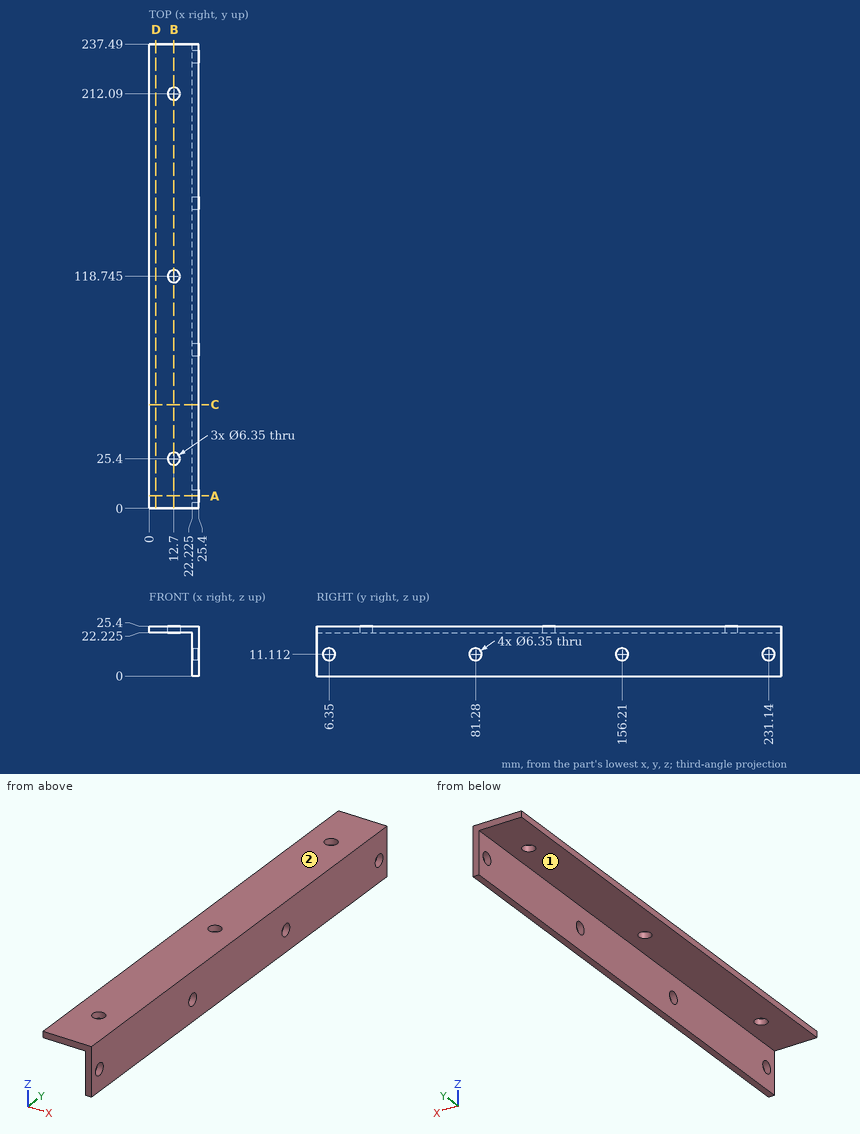
Verification items for this drawing (mm, ordinates from the low corner). A direction names the side the tool comes from. Coordinates: 2 decimals unless noted, no trailing zeros. Write each loop counter-clockwise with the first axis right and the second up, starting at its lowest first coordinate (ties: lowest second). Pieces come first, ordered by that corner, then holes. Notation, with made-up numbers: (-36, -17.75) -> (-18, -17.75) arc R8 ccw to (-18, -3.75) -> close; hole circle Ø10 at (4.5, -13). An arc over 180 degrees is marked (long way). One line per item, written item: value. Start each with the question number.
Q1. Cross-section at B-B on x = 12.7. Enter the section's corners in (y, z) (1 decimal).
Q2. Cross-section at D-D on x = 3.5. Enter the section's corners in (y, z) (1 decimal).
Q3. Access from +Z, -Z, +X, -X, +Y, -Y to the whole of each face (thin tool, end or side, straight path). Record for the marked faces 1 and 2.
Q4. Go/stop test with flat-tipped pins: P1, Ø12, axis at y = 142.5, z = 21, coming from the -X side; P2, Ø10, axis at y = 81.28, z = 11.11, coming from the -X side (1 decimal); P3, Ø1.5, axis at x = 6, y = 48.5, coming from the -Z side (1 decimal). Record where each tip stops, or that it passes through.
Q5. Thickness scan on L1, parallel to Y at x = 12.7, z = 23.85 (1 decimal); L2, parallel to Z at x = 24.05, y = 156.21; L3, parallel to X at y = 62, z = 14.25 (1 decimal). Record the ranges inside material, lowest first. Write a range as from..to.
Q6. Cross-section at A-A on y = 6.35. Enter the section's corners in (x, z) (1 decimal), and give its area (3 significant figures).
Q7. Cross-section at C-C on y = 53. Enter the section's corners in (x, z) (1 decimal), and give its area (3 significant figures).
Checked values:
1. outline: (0, 22.2) -> (22.2, 22.2) -> (22.2, 25.4) -> (0, 25.4) -> close; (28.6, 22.2) -> (115.6, 22.2) -> (115.6, 25.4) -> (28.6, 25.4) -> close; (121.9, 22.2) -> (208.9, 22.2) -> (208.9, 25.4) -> (121.9, 25.4) -> close; (215.3, 22.2) -> (237.5, 22.2) -> (237.5, 25.4) -> (215.3, 25.4) -> close
2. outline: (0, 22.2) -> (237.5, 22.2) -> (237.5, 25.4) -> (0, 25.4) -> close
3. face 1: -Z, -X, +Y, -Y
3. face 2: +Z, +X, -X, +Y, -Y
4. P1: stops at x = 0
4. P2: stops at x = 22.2
4. P3: stops at z = 22.2
5. L1: y = 0..22.2, 28.6..115.6, 121.9..208.9, 215.3..237.5
5. L2: z = 0..7.94, 14.29..25.4
5. L3: x = 22.2..25.4
6. outline: (0, 22.2) -> (22.2, 22.2) -> (22.2, 14.3) -> (25.4, 14.3) -> (25.4, 25.4) -> (0, 25.4) -> close; (22.2, 0) -> (25.4, 0) -> (25.4, 7.9) -> (22.2, 7.9) -> close
6. area: 131 mm²
7. outline: (0, 22.2) -> (22.2, 22.2) -> (22.2, 0) -> (25.4, 0) -> (25.4, 25.4) -> (0, 25.4) -> close
7. area: 151 mm²
